from build123d import *

# Parameters (mm, degrees)
PAD_DEPTH    = 5
PAD001_DEPTH = 5
PAD002_DEPTH = 5


with BuildPart() as part:
    # Sketch → Pad (new body)
    with BuildSketch(Plane.XY):
        Polygon((-3.47, -3.5), (3.47, -3.5), (3.47, -6.3), (9.128033, 3.5), (3.47, 3.5), (-3.47, 3.5), (-9.128033, 3.5), (-3.47, -6.3), align=None)
    extrude(amount=PAD_DEPTH)

    # Sketch001 (on Face9 of Pad) → Pad001 (join)
    with BuildSketch(Plane(origin=(0, 0, 0), x_dir=(1, 0, 0), z_dir=(0, 0, -1))):
        Polygon((-3.47, 6.299921), (-9.128033, -3.500079), (-3.47, -3.500079), align=None)
        Polygon((3.47, 6.299921), (9.128033, -3.500079), (3.47, -3.500079), align=None)
    extrude(amount=PAD001_DEPTH)

    # Sketch002 (on Face5 of Pad001) → Pad002 (join)
    with BuildSketch(Plane.XY.offset(5)):
        Polygon((-9.128033, 3.500297), (-3.47, -6.299703), (-3.47, 3.500297), align=None)
        Polygon((3.47, -6.299703), (3.47, 3.500297), (9.128033, 3.500297), align=None)
    extrude(amount=PAD002_DEPTH)


solid = part.part
Read the model definition and answer for the solid it produces. Units are mm, in the model's axes. A direction names the side the tool comes from. Coordinates: 2 decimals unless noted, no trailing zeros. Write each loop counter-clockwise with the first axis right and the second up, starting at its lowest first coordinate (ties: lowest second). Pieces come first, ordered by that corner, then holes. Notation, with made-up numbers: (20, 47) -> (63, 47) arc R28 ccw to (63, 80) -> close; hole circle Ø10 at (-34, 30.25). An arc over 180 degrees is marked (long way). Return JSON: item names as keys, results as strings.
(1) For a pull along X with two mould halves and no side action, classify faces 1 (the flat face through (-5, 1, 10)), 2 (the flat face through (6.26, -1.47, 2.46)), 3 (the flat face through (-3.47, -4, 2)), 4 (the flat face through (-6.26, -1.47, -2.46)) as pulls with the +X half, pulls with the -X half, needs draft (parallel to the pull), parting line crosses it, or undercut.
Answers below:
{"face 1": "needs draft", "face 2": "pulls with the +X half", "face 3": "undercut", "face 4": "pulls with the -X half"}
(2) The part is cut by section A-A on z = -0.25. Give the vertices of the cut face in (x, y).
Answers below:
{"outline": "(-9.13, 3.5) -> (-3.47, -6.3) -> (-3.47, 3.5) -> close; (3.47, -6.3) -> (9.13, 3.5) -> (3.47, 3.5) -> close"}
(3) Each of these flat-tipped pins is pushed along its axis until it touches: P1, Ø5, axis at y = -3.5, z = 8, coming from the -X side; P2, Ø4, axis at x = 1, z = 3.5, coming from the -Y side; P3, Ø1.5, axis at y = 2, z = 5, coming from the -X side (3 decimals); P4, Ø1, axis at x = -7, y = -2.5, coming from the -Z side. Where does it stop, or does it pass through?
Answers below:
{"P1": "x = -6.53", "P2": "y = -3.5", "P3": "x = -8.695", "P4": "through"}
(4) Consider line 1 along Y through (x, z) = (-2.25, 0.25); line 2 along Z through (x, y) = (1.5, -2); line 3 along X through (y, z) = (2.25, 7). Determine where each line is inside the solid, lowest interval first. Write a range as from..to.
Answers below:
{"line 1": "-3.5..3.5", "line 2": "0..5", "line 3": "-8.41..-3.47, 3.47..8.41"}
(5) Which of the six approach directions +Z, -Z, +X, -X, +Y, -Y give full straight-line access (tool end or side, diameter ignored) to faces 5 (the flat face through (3.47, -4, 2)), 6 (the flat face through (-6, 3.5, -2)), 7 (the flat face through (0, -3.5, 2)), 8 (the flat face through (0, 0, 0)), 9 (the flat face through (0, 0, 5))?
Answers below:
{"face 5": "-Y", "face 6": "+Z, -Z, +X, -X, +Y", "face 7": "+Z, -Z, -Y", "face 8": "-Z, +Y, -Y", "face 9": "+Z, +Y, -Y"}
